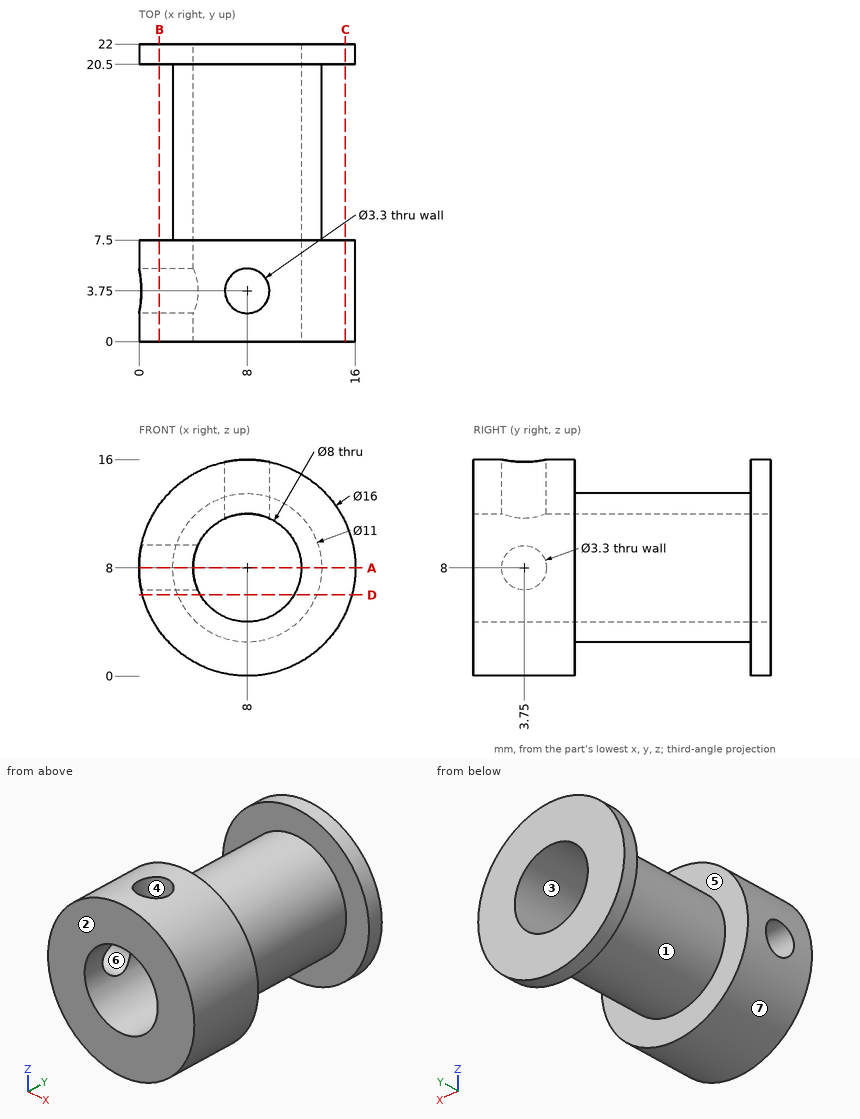
Verification items for this drawing (mm, ordinates from the low corner). A direction names the side the tool comes from. Round coordinates to 2 decimals unless told otherwise and drop trailing zeros. Write each loop counter-clockwise with the first axis right and the second up, starting at its lowest first coordinate (ties: lowest second). Pieces come first, ordered by that corner, then holes. Notation, with made-up numbers: M 6.25,1.5 L 13.25,1.5 A6 cw 13.25,6.5 Z; hole C 53,19 d4. An arc over 180 degrees is marked long. Write item = value, one per line. Start each with the question number.
1. Gauge pin test, flat ends, axial feed: pin 1 (4 mm diameter, centred on x = 3, y = 6, fed in from -Z); pin 2 (5 mm diameter, centred on y = 5.5, z = 2.5, fed in from -X); pin 3 (1.5 mm diameter, centred on x = 4.5, y = 15, fed in from +Z). Record the tip position at first contact, or that the pin passes through.
2. Section check D-D, the plane z = 6. Record the cut outline in (x, y).
3. Tool access check on the marked faces 4, 5, 6 and 7. Record the directions out of +Z, -Z, +X, -X, +Y, -Y that give a thin tool (end or side, any length) a straight path to the whole face; none if there is none.
4. Release check for a two-part mould opening along Z. For the marked faces 1, 2 and 3 record: pulls with the +Z half, pulls with the -Z half, needs draft (parallel to the pull), parting line crosses it, or undercut.
5. Section check B-B, the plane x = 1.5. Record the cut outline in (y, z).
6. Section check C-C, the plane x = 15.25. Record the cut outline in (y, z).
7. Scan lines: line 1 (Y direction, x = 11, z = 2); line 2 (Z direction, x = 8, y = 8.75); line 3 (Z direction, x = 5.5, y = 19.5). Record each from-to range of solid material in increasing order. Write a range as [from, to].
8. Section check A-A, the plane z = 8. Record the cut outline in (x, y).
Results found:
q1.pin_1 = 0.58
q1.pin_2 = 0.58
q1.pin_3 = 12.76
q2.outline = M 0.25,0 L 4.54,0 L 4.54,22 L 0.25,22 L 0.25,20.5 L 2.88,20.5 L 2.88,7.5 L 0.25,7.5 Z; M 11.46,0 L 15.75,0 L 15.75,7.5 L 13.12,7.5 L 13.12,20.5 L 15.75,20.5 L 15.75,22 L 11.46,22 Z
q3.face_4 = +Z
q3.face_5 = none
q3.face_6 = -X
q3.face_7 = +Y, -Y
q4.face_1 = parting line crosses it
q4.face_2 = needs draft
q4.face_3 = undercut
q5.outline = M 0,3.34 L 7.5,3.34 L 7.5,12.66 L 0,12.66 Z; M 20.5,3.34 L 22,3.34 L 22,12.66 L 20.5,12.66 Z; hole C 3.75,8 d3.3
q6.outline = M 0,4.62 L 7.5,4.62 L 7.5,11.38 L 0,11.38 Z; M 20.5,4.62 L 22,4.62 L 22,11.38 L 20.5,11.38 Z
q7.line_1 = [0, 7.5], [20.5, 22]
q7.line_2 = [2.5, 4], [12, 13.5]
q7.line_3 = [3.1, 4.88], [11.12, 12.9]
q8.outline = M 0,0 L 4,0 L 4,2.1 L 0,2.1 Z; M 0,5.4 L 4,5.4 L 4,22 L 0,22 L 0,20.5 L 2.5,20.5 L 2.5,7.5 L 0,7.5 Z; M 12,0 L 16,0 L 16,7.5 L 13.5,7.5 L 13.5,20.5 L 16,20.5 L 16,22 L 12,22 Z
